from build123d import *

# Parameters (mm, degrees)
F0_W     = 100
F0_H     = 100
F1_DEPTH = 4
F2_R     = 24.680496
F3_DEPTH = 25
F4_R     = 5
F5_DEPTH = 25
F6_R     = 10.957285
F7_DEPTH = 25
F8_R     = 1
F9_DEPTH = 4.001


with BuildPart() as f1:
    # F0 (on Front) → F1 (new body)
    with BuildSketch(Plane.XZ):
        Rectangle(F0_W, F0_H)
    extrude(amount=F1_DEPTH)

    # F2 (on face) → F3 (cut)
    with BuildSketch(Plane.XZ.offset(4)):
        Circle(F2_R)
    extrude(amount=-F3_DEPTH, mode=Mode.SUBTRACT)

    # F4 (on face) → F5 (cut)
    with BuildSketch(Plane.XZ.offset(4)):
        with Locations((31.545788, 33.773698)):
            Circle(F4_R)
    extrude(amount=-F5_DEPTH, mode=Mode.SUBTRACT)

    # F6 (on face) → F7 (cut)
    with BuildSketch(Plane.XZ.offset(4)):
        with Locations((-30.745968, 32.870423)):
            Circle(F6_R)
    extrude(amount=-F7_DEPTH, mode=Mode.SUBTRACT)

    # F8 (on face) → F9 (cut, through all)
    with BuildSketch(Plane.XZ.offset(4)):
        with Locations((0, 35)):
            Circle(F8_R)
    extrude(amount=-F9_DEPTH, mode=Mode.SUBTRACT)


solid = f1.part
Part model, mm, in its own coordinate system. Give positions to 0.01 mm unless a question says otherwise; leave off trailing zeros. Loops run counter-clockwise (first coordinate to the right, second up) from the corner with the lowest first, then second, coordinate; pieces in that order, holes last. Notation, with made-up numbers: M 54,22 L 74,22 A8 ccw 74,32 Z; hole C 15,57 d10. An arc over 180 degrees is marked long. Put each result on its own line as item: value. Start each with the question number.
1) Saw through at A-A (z = 0). List the corners of the cut face in (x, y).
2) Saw through at C-C (y = -1.45). List the corners of the cut face in (x, z).
3) Pull direction Z, two halves, no side cores. Call faces 1 (the flat face through (-1, -2, 50)), 2 (the flat face through (-23, 0, -10)), 3 (the cylindrical face through (-5.35, -2.028, -24.094)): +Z half, -Z half, draft (parallel to the pull), parting line (faces both ways), or undercut.
4) Probe probe 1 along Z at (x, y) = (0, -1.9); probe 2 along Z at (x, y) = (-19, -2.1); probe 3 along Z at (x, y) = (29.5, -2.85). List the from-to ranges inside material, lowest first.
5) Saw through at B-B (x = 28). List the corners of the cut face in (y, z), then the cut area to 3 significant figures.
6) Flat gauge pin, fed straight in: pin 1 (9 mm diameter, centred on x = 31.55, z = 33.77, fed in from -Y). Where does the tip first touch, or does it go through?
Numbers:
1. outline: M -50,-4 L -24.68,-4 L -24.68,0 L -50,0 Z; M 24.68,-4 L 50,-4 L 50,0 L 24.68,0 Z
2. outline: M -50,-50 L 50,-50 L 50,50 L -50,50 Z; hole C -30.75,32.87 d21.91; hole C 0,0 d49.36; hole C 0,35 d2; hole C 31.55,33.77 d10
3. face 1: +Z half
3. face 2: draft
3. face 3: undercut
4. probe 1: -50 to -24.68, 24.68 to 34, 36 to 50
4. probe 2: -50 to -15.75, 15.75 to 50
4. probe 3: -50 to 29.21, 38.34 to 50
5. outline: M -4,-50 L 0,-50 L 0,30.25 L -4,30.25 Z; M -4,37.3 L 0,37.3 L 0,50 L -4,50 Z
5. area: 372 mm^2
6. pin 1: through
